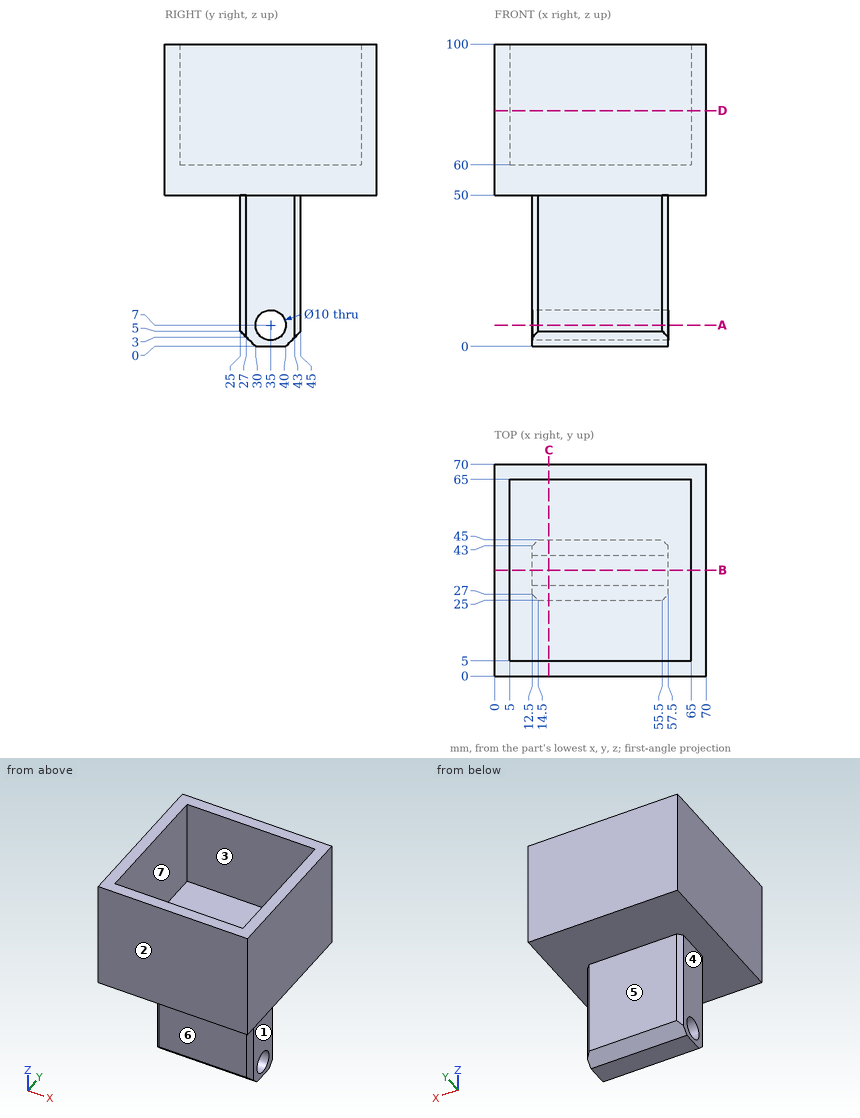
Study the drawing (mm; zero at the part's minimum x, y, z) and answer. A direction names the side the tool comes from. Give positions to 0.01 mm unless a question says otherwise; leave off trailing zeros. Order: outer loops, then holes, each group sorted by start corner. A loop starts at its lowest first (then second) coordinate and runs counter-clockwise, first axis right, second up.
1) Find section C-C on x = 18. Write down the section's boundary in (y, z).
Reported:
outline: (0, 50) - (25, 50) - (25, 5) - (30, 0) - (40, 0) - (45, 5) - (45, 50) - (70, 50) - (70, 100) - (65, 100) - (65, 60) - (5, 60) - (5, 100) - (0, 100) - close; hole circle Ø10 at (35, 7)
2) Given P1, Ø10, axis at x = 54, y = 36, coming from the +Z side; P2, Ø10, axis at y = 26, z = 23, coming from the -X side; P3, Ø20.5, axis at x = 29.5, z = 36, coming from the +Y side, each flat-ended and moving along its own axis, determine where each tip first touches the part or whether it passes through.
Reported:
P1: stops at z = 60
P2: stops at x = 12.5
P3: stops at y = 45
3) Find section D-D on z = 78. Write down the section's boundary in (x, y), then the cut area to 3 significant figures.
Reported:
outline: (0, 0) - (70, 0) - (70, 70) - (0, 70) - close; hole (5, 5) - (65, 5) - (65, 65) - (5, 65) - close
area: 1,300 mm2
4) Determine the mould class of the marked faces 1, 2 and 3 for opening direction Y: pulls with the +Y half, pulls with the -Y half, needs draft (parallel to the pull), parting line crosses it, or undercut.
Reported:
face 1: needs draft
face 2: pulls with the -Y half
face 3: undercut
5) Consider line 1 along X through (y, z) = (37, 85); line 2 along Z through (x, y) = (35, 35). Determine where each line is inside the solid, lowest interval first.
Reported:
line 1: x = 0 to 5, 65 to 70
line 2: z = 0 to 2, 12 to 60
6) Find section B-B on y = 35. Write down the section's boundary in (x, z), then the cut area to 3 significant figures.
Reported:
outline: (0, 50) - (12.5, 50) - (12.5, 12) - (57.5, 12) - (57.5, 50) - (70, 50) - (70, 100) - (65, 100) - (65, 60) - (5, 60) - (5, 100) - (0, 100) - close; (12.5, 0) - (57.5, 0) - (57.5, 2) - (12.5, 2) - close
area: 2,900 mm2
7) Find section A-A on z = 7. Write down the section's boundary in (x, y).
Reported:
outline: (12.5, 27) - (14.5, 25) - (55.5, 25) - (57.5, 27) - (57.5, 30) - (12.5, 30) - close; (12.5, 40) - (57.5, 40) - (57.5, 43) - (55.5, 45) - (14.5, 45) - (12.5, 43) - close
8) For the marked faces 4, 5, 6 and 7, determine the directions among +Z, -Z, +X, -X, +Y, -Y from which every point of the face is accessible in a straight line to the end or side of a thin tool.
Reported:
face 4: -Z, -X, +Y, -Y
face 5: -Z, +X, -X, +Y
face 6: -Z, +X, -X, -Y
face 7: +Z
